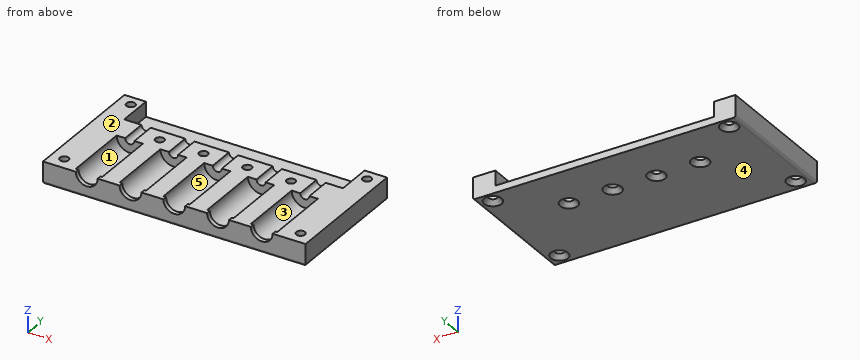
```python
from build123d import *

# Parameters (mm, degrees)
F0_W      = 60
F0_H      = 25
F1_DEPTH  = 5
F2_R      = 2.5
F3_DEPTH  = 10
F5_R      = 3
F6_DEPTH  = 15
F7_R      = 1.05
F8_DEPTH  = 29
F9_W      = 50
F9_H      = 3.4154356362
F10_DEPTH = 3
F11_DEPTH = 5
F12_R     = 0.5
F14_R     = 1
F13_R     = 1
F15_DEPTH = 5.001
F16_R     = 1
F17_DEPTH = 5.001
F18_SIZE  = 1


with BuildPart() as f1:
    # F0 (on Top) → F1 (new body)
    with BuildSketch(Plane.XY):
        with Locations((-2.9453901201, -7.2920476746)):
            Rectangle(F0_W, F0_H)
    extrude(amount=F1_DEPTH)

    # F2 (on face) → F3 (cut)
    with BuildSketch(Plane.XZ.offset(19.7920476746)):
        with Locations((-22.9453901201, 5)):
            Circle(F2_R)
        with Locations((-12.9453901201, 5)):
            Circle(F2_R)
        with Locations((-2.9453901201, 5)):
            Circle(F2_R)
        with Locations((7.0546098799, 5)):
            Circle(F2_R)
        with Locations((17.0546098799, 5)):
            Circle(F2_R)
    extrude(amount=-F3_DEPTH, mode=Mode.SUBTRACT)

    # F5 (on offset) → F6 (cut)
    with BuildSketch(Plane.XZ.offset(18.7920476746)):
        with Locations((-23.0476632714, 5.0127296709)):
            Circle(F5_R)
        with Locations((-13.0476632714, 5.0127296709)):
            Circle(F5_R)
        with Locations((-3.0476632714, 5.0127296709)):
            Circle(F5_R)
        with Locations((6.9523367286, 5.0127296709)):
            Circle(F5_R)
        with Locations((16.9523367286, 5.0127296709)):
            Circle(F5_R)
    extrude(amount=-F6_DEPTH, mode=Mode.SUBTRACT)

    # F7 (on face) → F8 (cut)
    with BuildSketch(Plane.XZ.offset(3.7920476746)):
        with Locations((-23.0476632714, 5.0127296709)):
            Circle(F7_R)
        with Locations((-13.0476632714, 5.0127296709)):
            Circle(F7_R)
        with Locations((-3.0476632714, 5.0127296709)):
            Circle(F7_R)
        with Locations((6.9523367286, 5.0127296709)):
            Circle(F7_R)
        with Locations((16.9523367286, 5.0127296709)):
            Circle(F7_R)
    extrude(amount=-F8_DEPTH, mode=Mode.SUBTRACT)

    # F9 (on face) → F10 (cut)
    with BuildSketch(Plane(origin=(0, 5.2079523254, 0), x_dir=(-1, 0, 0), z_dir=(0, 1, 0))):
        with Locations((3.0476632714, 3.2922821819)):
            Rectangle(F9_W, F9_H)
    extrude(amount=-F10_DEPTH, mode=Mode.SUBTRACT)

    # F11 (add): a face of the model
    f11_faces = [f1.faces().sort_by_distance(p)[0] for p in [
        (-2.8102387692, 5.2079523254, 1.4530193808),
    ]]
    extrude(f11_faces, amount=F11_DEPTH)

    # F12
    f12_edges = [f1.edges().sort_by_distance(p)[0] for p in [
        (27.05461, -4.792048, 0),
        (-2.94539, -19.792048, 0),
        (-32.94539, -4.792048, 0),
    ]]
    fillet(f12_edges, radius=F12_R)

    # F14 (on face) + F13 (on face) → F15 (cut, through all)
    with BuildSketch(Plane(origin=(0, 0, 0), x_dir=(1, 0, 0), z_dir=(0, 0, -1))):
        with Locations((-29.9453901201, -7.7079523254)):
            Circle(F14_R)
        with Locations((24.0546098799, -7.7079523254)):
            Circle(F14_R)
    with BuildSketch(Plane(origin=(0, 0, 0), x_dir=(1, 0, 0), z_dir=(0, 0, -1))):
        with Locations((-29.9453901201, 16.7920476746)):
            Circle(F13_R)
        with Locations((24.0546098799, 16.7920476746)):
            Circle(F13_R)
    extrude(amount=-F15_DEPTH, mode=Mode.SUBTRACT)

    # F16 (on face) → F17 (cut, through all)
    with BuildSketch(Plane.XY.offset(5)):
        with Locations((11.9524138955, -0.7920476746)):
            Circle(F16_R)
        with Locations((1.9524138955, -0.7920476746)):
            Circle(F16_R)
        with Locations((-8.0475861045, -0.7920476746)):
            Circle(F16_R)
        with Locations((-18.0475861045, -0.7920476746)):
            Circle(F16_R)
    extrude(amount=-F17_DEPTH, mode=Mode.SUBTRACT)

    # F18
    f18_edges = [f1.edges().sort_by_distance(p)[0] for p in [
        (23.05461, 7.707952, 0),
        (10.952414, -0.792048, 0),
        (23.05461, -16.792048, 0),
        (0.952414, -0.792048, 0),
        (-9.047586, -0.792048, 0),
        (-19.047586, -0.792048, 0),
        (-30.94539, 7.707952, 0),
        (-30.94539, -16.792048, 0),
    ]]
    chamfer(f18_edges, length=F18_SIZE)


solid = f1.part
```
Input: part model. Units: mm. Frame: model coordinates. Face numbers are marked on the shaded views. A direction names the side the tool comes from. Coordinates: 2 decimals unless noted, no trailing zeros. Loops run counter-clockwise (first coordinate to the right, second up) from the corner with the lowest first, then second, coordinate; pieces in that order, holes last.
Q1. Line query: line 1 along Y through (x, z) = (-30, 1.1); line 2 along X through (y, z) = (-8.5, 3.6); line 3 along Y through (x, z) = (-21, 2.9). Output: solid intervals per line, ascending.
Results are:
line 1: y = -19.79 to -17.79, -15.79 to 6.71, 8.71 to 10.21
line 2: x = -32.95 to -25.69, -20.4 to -15.69, -10.4 to -5.69, -0.4 to 4.31, 9.6 to 14.31, 19.6 to 27.05
line 3: y = -19.79 to -18.79, -3.79 to 2.21
Q2. Section C-C, the plane z = 3.15. Give the number of separate pieces and of enclosed holes in the cut face, and give its area (3 significant figures).
Results are:
separate pieces: 1
enclosed holes: 8
area: 1,010 mm2
Q3. Section A-A, the plane y = -9. Return the cut outline in (x, z).
Results are:
outline: (-32.95, 0.5) arc R0.5 ccw to (-32.45, 0) - (26.55, 0) arc R0.5 ccw to (27.05, 0.5) - (27.05, 5) - (19.95, 5) arc R3 cw to (13.95, 5) - (9.95, 5) arc R3 cw to (3.95, 5) - (-0.05, 5) arc R3 cw to (-6.05, 5) - (-10.05, 5) arc R3 cw to (-16.05, 5) - (-20.05, 5) arc R3 cw to (-26.05, 5) - (-32.95, 5) - close
Q4. Mould query, pull axis X, two halves, no side actions, for the marked faces 1, 2 and 3. Classes: +X half, -X half, draft (parallel to the pull), parting line (faces both ways), or undercut.
Results are:
face 1: undercut
face 2: draft
face 3: undercut
Q5. Set-up query: the marked faces 4 and 5. Return all of +Z, -Z, +X, -X, +Y, -Y with unobstructed straight access to the full face (end or side cutting, diameter ignored); none if empty.
Results are:
face 4: -Z, +X, -X, +Y, -Y
face 5: +Z
Q6. Section B-B, the plane x = 17. Return the cut outline in (y, z).
Results are:
outline: (-19.79, 0.5) arc R0.5 ccw to (-19.29, 0) - (10.21, 0) - (10.21, 1.58) - (2.21, 1.58) - (2.21, 3.96) - (-3.79, 3.96) - (-3.79, 2.01) - (-18.79, 2.01) - (-18.79, 2.5) - (-19.79, 2.5) - close
Q7. Contact query for flat-ended pins moving along their axis: pin 1 (4 mm diameter, centred on x = -5.5, y = 5, fed in from +Z); pin 2 (2.5 mm diameter, centred on x = -12, z = 4, fed in from +Y); pin 3 (1.6 mm diameter, centred on x = -29.95, y = -16.79, fed in from +Z); pin 4 (1 mm diameter, centred on x = 18.5, y = -16, fed in from +Z). Output: stop coordinate, or through.
Results are:
pin 1: stops at z = 1.58
pin 2: stops at y = 2.21
pin 3: passes through
pin 4: stops at z = 2.82
